```python
from build123d import *

# Parameters (mm, degrees)
F0_W     = 50
F0_H     = 50
F0_W_2   = 41
F0_H_2   = 40
F1_DEPTH = 47.5
F2_DEPTH = 45


# Not quite as in the source:
# - a feature names something its author has since deleted; it is built from what else it names


with BuildPart() as f1:
    # F0 (on Front) → F1 (new body)
    with BuildSketch(Plane.XZ):
        with Locations((-14.9696101435, 1.412372324)):
            Rectangle(F0_W, F0_H)
        with Locations((-14.9696101435, 1.912372324)):
            Rectangle(F0_W_2, F0_H_2, mode=Mode.SUBTRACT)
        with Locations((-14.9696101435, 1.912372324)):
            Rectangle(F0_W_2, F0_H_2)
    extrude(amount=F1_DEPTH)

    # F0 (on Front) → F2 (cut)
    with BuildSketch(Plane.XZ):
        with Locations((-14.9696101435, 1.912372324)):
            Rectangle(F0_W_2, F0_H_2)
    extrude(amount=F2_DEPTH, mode=Mode.SUBTRACT)


solid = f1.part
```
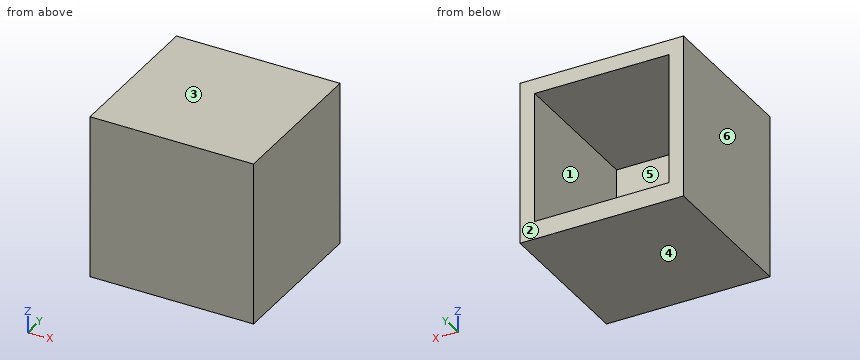
Source: CAD feature listing. Evaluate the final solid. Frame: model axes, mm. Face numbers are marked on the shaded views. A direction names the side the tool comes from. Give positions to 0.01 mm unless a question says otherwise; leave off trailing zeros. Order: outer loops, then holes, each group sorted by start corner. A loop starts at its lowest first (then second) coordinate and runs counter-clockwise, first axis right, second up.
(1) Section query B-B (z = -7). Return the cut outline in (x, y), plus the area to 3 significant figures.
(2) Section query C-C (y = -32). Return the cut outline in (x, z), plus the area to 3 significant figures.
(3) Pull-direction query (Z, two-part tool) for the marked faces 3, 4, 5 and 6; classes: +Z half, -Z half, draft (parallel to the pull), parting line (faces both ways), or undercut.
(4) Contact query for a flat-ended pin moving along its axis: P1, Ø20, axis at x = -8.5, z = 5.5, coming from the +Y side. Output: stop coordinate, or through.
(5) Access query for the marked faces 1 and 2. Directions: +Z, -Z, +X, -X, +Y, -Y. A direction counts if a zero-diameter tool reaches every point of the face in a straight line with its end or side. Return the directions, or none.
(6) Section query A-A (x = -26). Return the cut outline in (y, z), plus the area to 3 significant figures.
(7) Material intervals for line 1 along X through (y, z) = (-4, 15); line 2 along Z through (x, y) = (-25, -19.5); line 3 along Y through (x, z) = (-34, -7), sorted ascending.
Outcome:
1. outline: (-39.97, -47.5) - (10.03, -47.5) - (10.03, 0) - (5.53, 0) - (5.53, -45) - (-35.47, -45) - (-35.47, 0) - (-39.97, 0) - close
1. area: 530 mm2
2. outline: (-39.97, -23.59) - (10.03, -23.59) - (10.03, 26.41) - (-39.97, 26.41) - close; hole (-35.47, -18.09) - (5.53, -18.09) - (5.53, 21.91) - (-35.47, 21.91) - close
2. area: 860 mm2
3. face 3: +Z half
3. face 4: -Z half
3. face 5: undercut
3. face 6: draft
4. P1: stops at y = -45
5. face 1: +Y
5. face 2: +Z, -Z, +X, -X, +Y
6. outline: (-47.5, -23.59) - (0, -23.59) - (0, -18.09) - (-45, -18.09) - (-45, 21.91) - (0, 21.91) - (0, 26.41) - (-47.5, 26.41) - close
6. area: 575 mm2
7. line 1: x = -39.97 to -35.47, 5.53 to 10.03
7. line 2: z = -23.59 to -18.09, 21.91 to 26.41
7. line 3: y = -47.5 to -45
